Check sheet for the modelled part. Datum: model origin and axes. Units: mm. Face numbers are marked on the shaded views. A direction names the side the tool comes from. Coordinates: 2 decimals unless noted, no trailing zeros. Loops run counter-clockwise (first coordinate to the right, second up) from the corner with the lowest first, then second, coordinate; pieces in that order, holes last. Notation, with made-up numbers: (74.25, 59) - (132.25, 59) arc R26 ccw to (132.25, 80) - close; hole circle Ø3 at (18.25, 19). An arc over 180 degrees is marked (long way). Use a Markdown table: item, result. Add a question column.
1) Sectioned sample at B-B, the plane z = 12.25. Enter the section's corners in (x, y).
2) Sectioned sample at A-A, the plane z = 21. Enter the section's corners in (x, y) (3 decimals).
3) Draft check along X on the marked faces 3, 4 and 5. Enter one of: pulls with the +X half, pulls with the -X half, needs draft (parallel to the pull), parting line crosses it, or undercut.
4) Thickness scan on line 1 (Y direction, x = 0, z = 5.5); line 2 (Z direction, x = 12, y = -15); line 3 (Y direction, x = 0, z = 18.5) (3 decimals). Record the ranges inside material, lowest first.
5) Go/stop test with flat-tipped pins: P1, Ø10, axis at x = 18, z = 7.5, coming from the -Y side; P2, Ø4, axis at y = 8.5, z = 10, coming from the +X side; P3, Ø8, axis at x = -13.5, z = 4, coming from the +Y side; P4, Ø23, axis at x = 0, y = 0, coming from the +Z side. Record where each tip stops, or that it passes through.
6) Tool access check on the marked faces 1 and 2. Record the directions out of +Z, -Z, +X, -X, +Y, -Y that give a thin tool (end or side, any length) a straight path to the whole face; none if there is none.
from build123d import *

# Parameters (mm, degrees)
SKETCH1_R           = 25
BOSS_EXTRUDE1_DEPTH = 15
SKETCH2_R           = 16.855
BOSS_EXTRUDE2_DEPTH = 10
SKETCH3_R           = 12.7
CUT_EXTRUDE1_DEPTH  = 30


with BuildPart() as part:
    # Sketch1 → Boss-Extrude1 (new body)
    with BuildSketch(Plane.XY):
        Circle(SKETCH1_R)
    extrude(amount=BOSS_EXTRUDE1_DEPTH)

    # Sketch2 → Boss-Extrude2 (add)
    with BuildSketch(Plane.XY.offset(15)):
        Circle(SKETCH2_R)
    extrude(amount=BOSS_EXTRUDE2_DEPTH)

    # Sketch3 → Cut-Extrude1 (cut)
    with BuildSketch(Plane.XY.offset(25)):
        Circle(SKETCH3_R)
    extrude(amount=-CUT_EXTRUDE1_DEPTH, mode=Mode.SUBTRACT)

    # Sketch8 → Cut-Revolve13 (revolve, cut)
    with BuildSketch(Plane(origin=(0, 0, 0), x_dir=(0, 0, -1), z_dir=(1, 0, 0)), mode=Mode.PRIVATE) as cut_revolve13_sk:
        with BuildLine():
            Line((-15, 26.011262748), (-15, 24.311262748))
            ThreePointArc((-15, 24.311262748), (-7.5, 25.954168843), (0, 24.311262748))
            Line((0, 24.311262748), (0, 26.011262748))
            Line((0, 26.011262748), (-15, 26.011262748))
        make_face()
    revolve(cut_revolve13_sk.sketch.rotate(Axis((0, 0, 0), (0, 0, 1)), 90), axis=Axis((0, 0, 0), (0, 0, 1)), mode=Mode.SUBTRACT)


solid = part.part
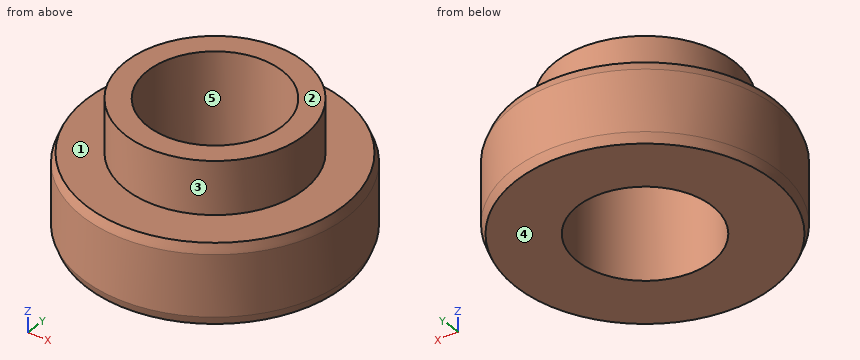
Solved:
| question | item | result |
|---|---|---|
| 1 | outline | circle Ø50 at (0, 0); hole circle Ø25.4 at (0, 0) |
| 2 | outline | circle Ø33.71 at (0, 0); hole circle Ø25.4 at (0, 0) |
| 3 | face 3 | parting line crosses it |
| 3 | face 4 | needs draft |
| 3 | face 5 | undercut |
| 4 | line 1 | y = -25 to -12.7, 12.7 to 25 |
| 4 | line 2 | z = 0 to 15 |
| 4 | line 3 | y = -16.855 to -12.7, 12.7 to 16.855 |
| 5 | P1 | stops at y = -21.35 |
| 5 | P2 | stops at x = 24.14 |
| 5 | P3 | stops at y = 23.12 |
| 5 | P4 | passes through |
| 6 | face 1 | +Z |
| 6 | face 2 | +Z, +X, -X, +Y, -Y |
